Part model, mm, in its own coordinate system. Face numbers are marked on the shaded views. A direction names the side the tool comes from. Give positions to 0.01 mm unless a question says otherwise; leave off trailing zeros. Order: outer loops, then holes, each group sorted by start corner. A loop starts at its lowest first (then second) coordinate and runs counter-clockwise, first axis right, second up. Notation, with made-up numbers: M -16,13.5 L 24,13.5 A30 ccw 24,49.5 Z; hole C -22,69 d6. An arc over 180 degrees is marked long. Answer as a JSON object with one key per item and string values.
from build123d import *

# Parameters (mm, degrees)
F0_W     = 72
F0_H     = 33
F1_DEPTH = 25
F2_T     = -3
F3_R     = 2.5
F3_W     = 3
F3_H     = 27
F4_DEPTH = 10


with BuildPart() as f1:
    # F0 (on Top) → F1 (new body)
    with BuildSketch(Plane.XY):
        Rectangle(F0_W, F0_H)
    extrude(amount=F1_DEPTH)

    # F2
    f2_openings = [f1.faces().sort_by_distance(p)[0] for p in [
        (0, 0, 0),
    ]]
    offset(amount=F2_T, openings=f2_openings)

    # F3 (on face) → F4 (join)
    with BuildSketch(Plane(origin=(0, 0, 22), x_dir=(1, 0, 0), z_dir=(0, 0, -1))):
        Circle(F3_R)
        with Locations((-21.5, 0)):
            Rectangle(F3_W, F3_H)
        with Locations((21.5, 0)):
            Rectangle(F3_W, F3_H)
    extrude(amount=F4_DEPTH)


solid = f1.part
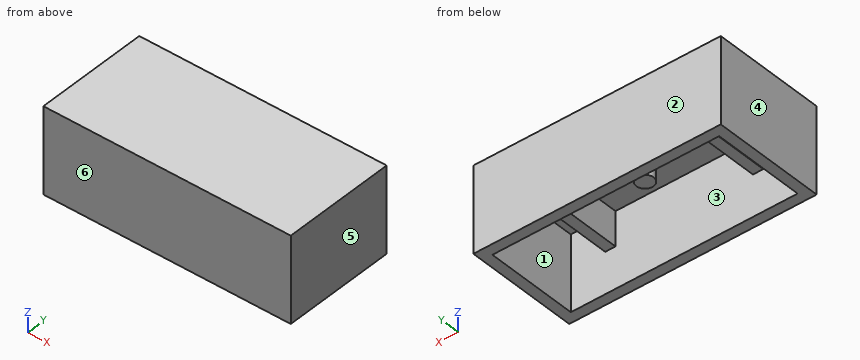
1. Pin check, flat tips, straight feed: P1, Ø5, axis at x = 14.5, y = 5, coming from the -Z side; P2, Ø1.5, axis at x = 1, y = 0, coming from the -Z side; P3, Ø5, axis at x = 3, y = 12.5, coming from the -Z side. Stop position of each tip, or through.
Worked answers:
{"P1": "stops at z = 22", "P2": "stops at z = 12", "P3": "stops at z = 0"}
2. Two-plate mould, pull along X, no slides. Class the marked faces 3, 4, 5 and 6: +X half, -X half, draft (parallel to the pull), parting line (faces both ways), or undercut.
Worked answers:
{"face 3": "undercut", "face 4": "-X half", "face 5": "+X half", "face 6": "draft"}
3. Which spindle directions (+Z, -Z, +X, -X, +Y, -Y) get a long thin tool onto all of the face, cutting with end or side? Do the marked faces 1 and 2. Say none if no direction does.
Worked answers:
{"face 1": "-Z", "face 2": "+Z, -Z, +X, -X, +Y"}
4. Cut at A-A on z = 12.75. Give the cut face in (x, y), plus the area to 3 significant figures.
Worked answers:
{"outline": "M -36,-16.5 L 36,-16.5 L 36,16.5 L -36,16.5 Z; C 0,0 d5; hole M -33,-13.5 L -23,-13.5 L -23,13.5 L -33,13.5 Z; hole M -20,-13.5 L 20,-13.5 L 20,13.5 L -20,13.5 Z; hole M 23,-13.5 L 33,-13.5 L 33,13.5 L 23,13.5 Z", "area": "776 mm^2"}
5. Cut at C-C on z = 9.5. Give the cut face in (x, y).
Worked answers:
{"outline": "M -36,-16.5 L 36,-16.5 L 36,16.5 L -36,16.5 Z; hole M -33,-13.5 L 33,-13.5 L 33,13.5 L -33,13.5 Z"}
6. Cut at B-B on x = 30. Give the cut face in (y, z).
Worked answers:
{"outline": "M -16.5,0 L -13.5,0 L -13.5,22 L 13.5,22 L 13.5,0 L 16.5,0 L 16.5,25 L -16.5,25 Z"}
7. Cut at D-D on y = 0. Give the cut face in (x, z).
Worked answers:
{"outline": "M -36,0 L -33,0 L -33,22 L -23,22 L -23,12 L -20,12 L -20,22 L -2.5,22 L -2.5,12 L 2.5,12 L 2.5,22 L 20,22 L 20,12 L 23,12 L 23,22 L 33,22 L 33,0 L 36,0 L 36,25 L -36,25 Z"}
8. Probe line 1 along X through (y, z) = (6, 20); line 2 along X through (y, z) = (-8, 2.25); line 3 along Y through (x, z) = (28.5, 19.75). List the from-to ranges inside material, lowest first.
Worked answers:
{"line 1": "x = -36 to -33, -23 to -20, 20 to 23, 33 to 36", "line 2": "x = -36 to -33, 33 to 36", "line 3": "y = -16.5 to -13.5, 13.5 to 16.5"}
